Source: CAD feature listing. Evaluate the final solid. Frame: model axes, mm. Give positions to 0.01 mm unless a question says otherwise; leave off trailing zeros. Order: outer loops, then holes, each group sorted by start corner. A loop starts at its lowest first (then second) coordinate and runs counter-clockwise, first axis right, second up. Notation, with made-up numbers: M 27,54.25 L 51,54.25 A10 cw 51,69.25 Z; hole C 10,54.5 d10. An arc over 180 degrees is marked long. Use CSV: the item, a comma, the result in double quotes. Start each with the question number.
Item 1: First-contact query: pin 1 (6.5 mm diameter, centred on x = -17.87, y = 15.79, fed in from +Z). Flat tip, straight axial feed; report the tip coordinate or a pass-through.
Item 2: Section query A-A on y = -18.5. Return loops of the section in (x, z), and give its area (3 significant figures).
Item 3: Section query B-B on z = 1.15. Return loops of the section in (x, y).
Item 4: Section query C-C on x = -14. Return loops of the section in (y, z), and give its area (3 significant figures).
Item 5: Section query D-D on y = -0.5. Return loops of the section in (x, z).
Item 6: Ray query, probe 1 along X at (y, z) = (14, 0.7); probe 2 along Y at (x, z) = (-14, 1.45); probe 3 along X at (y, z) = (15, 1). Return the intervals inside material, ascending. Write a range as from..to.
Autodesk Inventor part; units mm, degrees
ref_plane "YZ Plane" through (0, 0, 0) normal (1, 0, 0) x (0, 1, 0)
ref_plane "XZ Plane" through (0, 0, 0) normal (0, 1, 0) x (-1, 0, 0)
ref_plane "XY Plane" through (0, 0, 0) normal (0, 0, 1) x (1, 0, 0)
sketch "main" plane through (0, 0, 0) normal (0, 0, 1) x (1, 0, 0)
  circle A0 centre (-12.7091, -24.4332) radius 2.1844
  circle A1 centre (25.3909, -24.4332) radius 2.1844
  arc A2 (19.133, -23.3552) -> (31.7154, -23.8647) centre (25.3909, -24.4332) ccw
  arc A3 (-18.8897, -25.8904) -> (-7.3754, -20.9874) centre (-12.7091, -24.4332) ccw
  arc A4 (29.1539, 4.6304) -> (-24.0536, -3.989) centre (2.2439, 2.2114) ccw
  line L0 (29.1539, 4.6304) -> (31.7154, -23.8647)
  line L1 (-24.0536, -3.989) -> (-18.8897, -25.8904)
  arc A5 (22.6597, -1.0109) -> (-15.1169, -9.0043) centre (2.2439, 2.2114) ccw
  line L2 (19.133, -23.3552) -> (22.6597, -1.0109)
  line L3 (-7.3754, -20.9874) -> (-15.1169, -9.0043)
  circle A6 centre (-15.6258, 17.9972) radius 2.0955
  circle A7 centre (14.445, 22.6967) radius 2.0955
  point P0 (4.9022, -14.671)
  dimension "d0" = 12.7
  dimension "d1" = 12.7
  dimension "d2" = 6.35
  dimension "d5" = 4.191
  dimension "d6" = 23.8436
  dimension "d7" = 4.191
  dimension "d8" = 23.8436
sketch "Sketch1" plane through (0, 0, 0) normal (0, 0, 1) x (1, 0, 0)
  circle A0 centre (-14.953, -26.6446) radius 2.1844
  circle A1 centre (23.147, -26.6446) radius 2.1844
  arc A2 (16.8891, -25.5667) -> (29.4715, -26.0761) centre (23.147, -26.6446) ccw
  arc A3 (-21.1336, -28.1018) -> (-9.6193, -23.1988) centre (-14.953, -26.6446) ccw
  arc A4 (26.9101, 2.4189) -> (-26.2975, -6.2004) centre (0, 0) ccw
  line L0 (26.9101, 2.4189) -> (29.4715, -26.0761)
  line L1 (-26.2975, -6.2004) -> (-21.1336, -28.1018)
  arc A5 (20.4158, -3.2223) -> (-17.3608, -11.2157) centre (0, 0) ccw
  line L2 (16.8891, -25.5667) -> (20.4158, -3.2223)
  line L3 (-9.6193, -23.1988) -> (-17.3608, -11.2157)
  circle A6 centre (-17.8696, 15.7858) radius 2.0955
  circle A7 centre (12.2011, 20.4853) radius 2.0955
extrude "Extrusion1" add sketch "Sketch1" along normal blind 1.5875
properties part number "Reservoir Mount"
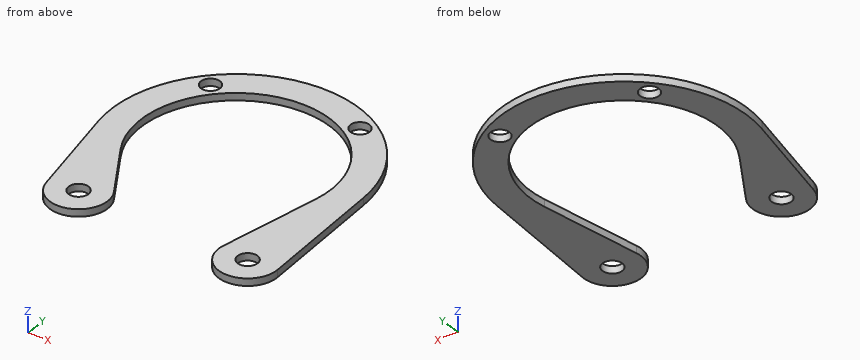
Verdict:
1,pin 1,"z = 1.59"
2,outline,"M -23.4,0 L -12.65,0 L -12.65,1.59 L -23.4,1.59 Z; M 18,0 L 28.79,0 L 28.79,1.59 L 18,1.59 Z"
2,area,"34.2 mm2"
3,outline,"M -26.3,-6.2 L -21.13,-28.1 A6.35 ccw long -9.62,-23.2 L -17.36,-11.22 A20.67 cw long 20.42,-3.22 L 16.89,-25.57 A6.35 ccw long 29.47,-26.08 L 26.91,2.42 A27.02 ccw long Z; hole C -17.87,15.79 d4.19; hole C -14.95,-26.64 d4.37; hole C 12.2,20.49 d4.19; hole C 23.15,-26.64 d4.37"
4,outline,"M -32.92,0 L -28.61,0 L -28.61,1.59 L -32.92,1.59 Z; M -24.68,0 L -16.42,0 L -16.42,1.59 L -24.68,1.59 Z; M 15.2,0 L 23.11,0 L 23.11,1.59 L 15.2,1.59 Z"
4,area,"32.5 mm2"
5,outline,"M -27.01,0 L -20.66,0 L -20.66,1.59 L -27.01,1.59 Z; M 20.66,0 L 27.17,0 L 27.17,1.59 L 20.66,1.59 Z"
6,probe 1,"-23.11..-18.97, -16.77..-15.2, 15.2..23.11"
6,probe 2,"-32.92..-28.61, -24.68..-16.42, 15.2..23.11"
6,probe 3,"-22.47..-19.81, -15.93..-14.22, 14.22..22.47"
